Geometry: final body of the model. Coordinates: model frame, mm. Face numbers are marked on the shaded views. A direction names the side the tool comes from. Give positions to 0.01 mm unless a question says otherwise; leave off trailing zeros. Write each loop counter-clockwise with the first axis right and the second up, starting at its lowest first coordinate (ties: lowest second). Pieces come first, ordered by that corner, then holes. Notation, with made-up numbers: M 85,-10 L 127,-10 A8 ccw 127,-1 Z; hole C 58,71.5 d3. An arc over 180 degrees is marked long. Answer as a JSON object with one key per item and string values.
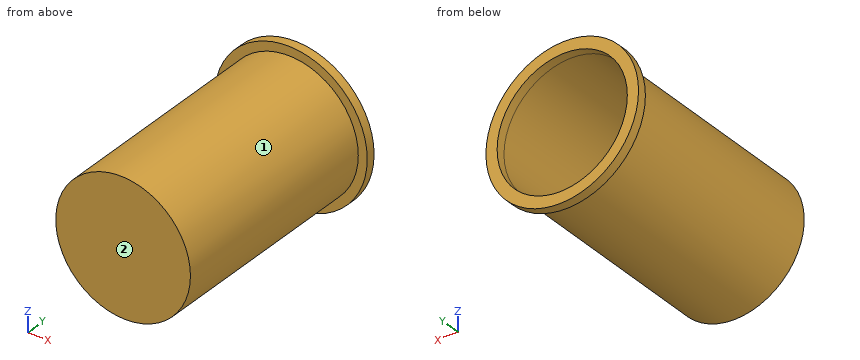
Autodesk Inventor part; units mm, degrees
ref_plane "YZ Plane" through (0, 0, 0) normal (1, 0, 0) x (0, 1, 0)
ref_plane "XZ Plane" through (0, 0, 0) normal (0, 1, 0) x (-1, 0, 0)
ref_plane "XY Plane" through (0, 0, 0) normal (0, 0, 1) x (1, 0, 0)
sketch "Sketch1" plane through (0, 0, 0) normal (0, 1, 0) x (-1, 0, 0)
  circle A0 centre (0, 0) radius 215.9
  circle A1 centre (0, 0) radius 184.15
  dimension "d0" = 431.8
  dimension "d1" = 368.3
extrude "Extrusion1" add sketch "Sketch1" along normal blind 25.4
sketch "Sketch2" plane through (0, 0, 0) normal (0, -1, 0) x (1, 0, 0)
  circle A0 centre (0, 0) radius 184.15
  circle A1 centre (0, 0) radius 190.5
  dimension "d4" = 381
extrude "Extrusion2" add sketch "Sketch2" along normal blind 609.6
sketch "Sketch3" plane through (0, -609.6, 0) normal (0, -1, 0) x (1, 0, 0)
  circle A0 centre (0, 0) radius 190.5
extrude "Extrusion3" add sketch "Sketch3" along normal blind 12.7
properties part number "Radiation Sheild 55K bottom"
1) Cut plane A-A on x = 0. Return loops of the section in (y, z).
Geometry check:
{"outline": "M -622.3,-190.5 L 0,-190.5 L 0,-215.9 L 25.4,-215.9 L 25.4,-184.15 L -609.6,-184.15 L -609.6,184.15 L 25.4,184.15 L 25.4,215.9 L 0,215.9 L 0,190.5 L -622.3,190.5 Z"}
2) Contact query for flat-ended pins moving along their axis: P1, Ø4, axis at x = -25.5, z = 46, coming from the +Y side; P2, Ø1, axis at x = -45.5, y = -446, coming from the +Z side; P3, Ø10, axis at y = -403.5, z = 57, coming from the +X side. Output: stop coordinate, or through.
Geometry check:
{"P1": "stops at y = -609.6", "P2": "stops at z = 185.11", "P3": "stops at x = 183.27"}
3) Set-up query: the marked faces 1 and 2. Return all of +Z, -Z, +X, -X, +Y, -Y with unobstructed straight access to the full face (end or side cutting, diameter ignored); none if empty.
Geometry check:
{"face 1": "-Y", "face 2": "+Z, -Z, +X, -X, -Y"}
4) Cut plane B-B on y = -416. Return loops of the section in (x, z).
Geometry check:
{"outline": "C 0,0 d381; hole C 0,0 d368.3"}
5) Cut plane C-C on z = -62. Return loops of the section in (x, y).
Geometry check:
{"outline": "M -206.81,0 L -180.13,0 L -180.13,-622.3 L 180.13,-622.3 L 180.13,0 L 206.81,0 L 206.81,25.4 L 173.4,25.4 L 173.4,-609.6 L -173.4,-609.6 L -173.4,25.4 L -206.81,25.4 Z"}
6) Line query: line 1 (Z direction, x = 0, y = 19); line 2 (Z direction, x = 0, y = -365); line 3 (Y direction, x = 24, z = -163.5). Output: solid intervals per line, ascending. Write a range as from..to.
Geometry check:
{"line 1": "z = -215.9..-184.15, 184.15..215.9", "line 2": "z = -190.5..-184.15, 184.15..190.5", "line 3": "y = -622.3..-609.6"}
